The model under review builds one solid part; all positions refer to its coordinate system, in mm. A direction names the side the tool comes from. Give positions to 0.01 mm unless a question says otherwise; leave off trailing zeros. Write each loop counter-clockwise with the first axis right and the second up, starting at its lowest first coordinate (ties: lowest second). Pieces come first, ordered by that corner, then holes. Notation, with made-up numbers: (-32.75, -20) -> (-6.75, -20) arc R22 cw to (-6.75, -2) -> close; hole circle Ø4 at (79.25, 16.5). An arc over 180 degrees is marked (long way). Use CSV: the item, a comma, the result in double quotes.
Autodesk Inventor part; units mm, degrees
ref_plane "YZ Plane" through (0, 0, 0) normal (1, 0, 0) x (0, 1, 0)
ref_plane "XZ Plane" through (0, 0, 0) normal (0, 1, 0) x (-1, 0, 0)
ref_plane "XY Plane" through (0, 0, 0) normal (0, 0, 1) x (1, 0, 0)
sketch "Sketch1" plane through (0, 0, 0) normal (0, 1, 0) x (-1, 0, 0)
  circle A0 centre (0, 0) radius 19.05
  dimension "d0" = 38.1
extrude "Extrusion1" add sketch "Sketch1" along normal blind 5.08
chamfer "Chamfer1" distance 8.89 distance2 5.08 1 edges at (19.05, 5.08, 0) measured on face at (-1.662, 5.08, -1.5197)
sketch "Sketch2" plane through (0, 5.08, 0) normal (0, 1, 0) x (1, 0, 0)
  circle A0 centre (0, 0) radius 19.05
extrude "Extrusion2" add sketch "Sketch2" along normal blind 5.08
chamfer "Chamfer2" distance 8.89 distance2 5.08 1 edges at (-19.05, 5.08, 0) measured on face at (15.8038, 5.08, 2.3301)
sketch "Sketch4" plane through (0, 10.16, 0) normal (0, 1, 0) x (1, 0, 0)
  circle A0 centre (0, 0) radius 2.794
  line L0 (0, 0) -> (-7.874, 0)
  line L1 (-7.874, 0) -> (-13.716, 0)
  line L2 (0, 0) -> (0, 7.874)
  line L3 (0, 0) -> (7.874, 0)
  line L4 (0, 0) -> (0, -7.874)
  circle A1 centre (0, -7.874) radius 1.397
  circle A2 centre (7.874, 0) radius 1.397
  circle A3 centre (0, 7.874) radius 1.397
  circle A4 centre (-7.874, 0) radius 1.397
  circle A5 centre (-13.716, 0) radius 1.397
  dimension "d28" = 5.588
  dimension "d29" = 7.874
  dimension "d30" = 5.842
  dimension "d31" = 7.874
  dimension "d32" = 7.874
  dimension "d33" = 7.874
  dimension "d34" = 2.794
  dimension "d35" = 2.794
  dimension "d36" = 2.794
  dimension "d37" = 2.794
  dimension "d38" = 2.794
  dimension "d15" = 7.874
  dimension "d16" = 5.842
  dimension "d17" = 5.588
  dimension "d18" = 2.794
  dimension "d19" = 2.794
  dimension "d20" = 7.874
  dimension "d21" = 7.874
  dimension "d22" = 7.874
  dimension "d23" = 2.794
  dimension "d24" = 2.794
  dimension "d25" = 2.794
extrude "Extrusion3" cut sketch "Sketch4" against normal blind 10.16
properties part number "LittleBigWheel v3"
Q1. Insertion check: pin 1 (6 mm diameter, centred on y = 4, z = 11, fed in from -X); pin 2 (5 mm diameter, centred on y = 6.5, z = -10, fed in from -X); pin 3 (1.5 mm diameter, centred on x = 1.5, y = 2, fed in from -Z). Each pin has a flat end and moves straight along its axis. Give the tip position at first contact, or say it passes through.
Derived:
pin 1,"stops at x = -13.75"
pin 2,"stops at x = -14.05"
pin 3,"stops at z = -16.8"
Q2. The part is to be moulded in two halves that separate along Y. For faces 1 (the conical face through (2.323, 4.762, 10.461)), 2 (the cylindrical face through (-0.18, 5.15, -9.26)), 3 (the flat face through (4, 10.16, 0)), say which applies: pulls with the +Y half, pulls with the -Y half, needs draft (parallel to the pull), parting line crosses it, or undercut.
Derived:
face 1,"undercut"
face 2,"needs draft"
face 3,"pulls with the +Y half"
Q3. Machinability: for faces 4 (the cylindrical face through (-0.18, 5.15, 6.49)), 5 (the conical face through (9.899, 5.398, 4.105)), which of the approach directions +Z, -Z, +X, -X, +Y, -Y give a long, thin tool a straight path to every point of the face, cutting with its end or side? Answer none if there is none.
Derived:
face 4,"+Y, -Y"
face 5,"none"
Q4. To check wall thickness, follow probe 1 along X at (y, z) = (6.5, 0); probe 2 along X at (y, z) = (3.25, -1); probe 3 along Z at (x, y) = (0, 3.5). State the ranges of each line that lie inside material, in increasing order.
Derived:
probe 1,"x = -12.32 to -9.27, -6.48 to -2.79, 2.79 to 6.48, 9.27 to 12.65"
probe 2,"x = -12.74 to -8.85, -6.9 to -2.61, 2.61 to 6.9, 8.85 to 13.33"
probe 3,"z = -12.93 to -9.27, -6.48 to -2.79, 2.79 to 6.48, 9.27 to 12.93"
Q5. Consider section C-C (y = 7.5). Write out the cut boundary in (x, z), then the cut area to 3 significant figures.
Derived:
outline,"(-14.34, -1.25) arc R14.4 ccw (long way) to (-14.34, 1.25) arc R1.4 cw (long way) to start; hole circle Ø2.79 at (-7.87, 0); hole circle Ø5.59 at (0, 0); hole circle Ø2.79 at (0, -7.87); hole circle Ø2.79 at (0, 7.87); hole circle Ø2.79 at (7.87, 0)"
area,"597 mm2"
Q6. Consider section A-A (z = 0). State how many separate pieces and enclosed holes the cut face has, then the cut area to 3 significant figures.
Derived:
separate pieces,"6"
enclosed holes,"0"
area,"166 mm2"
